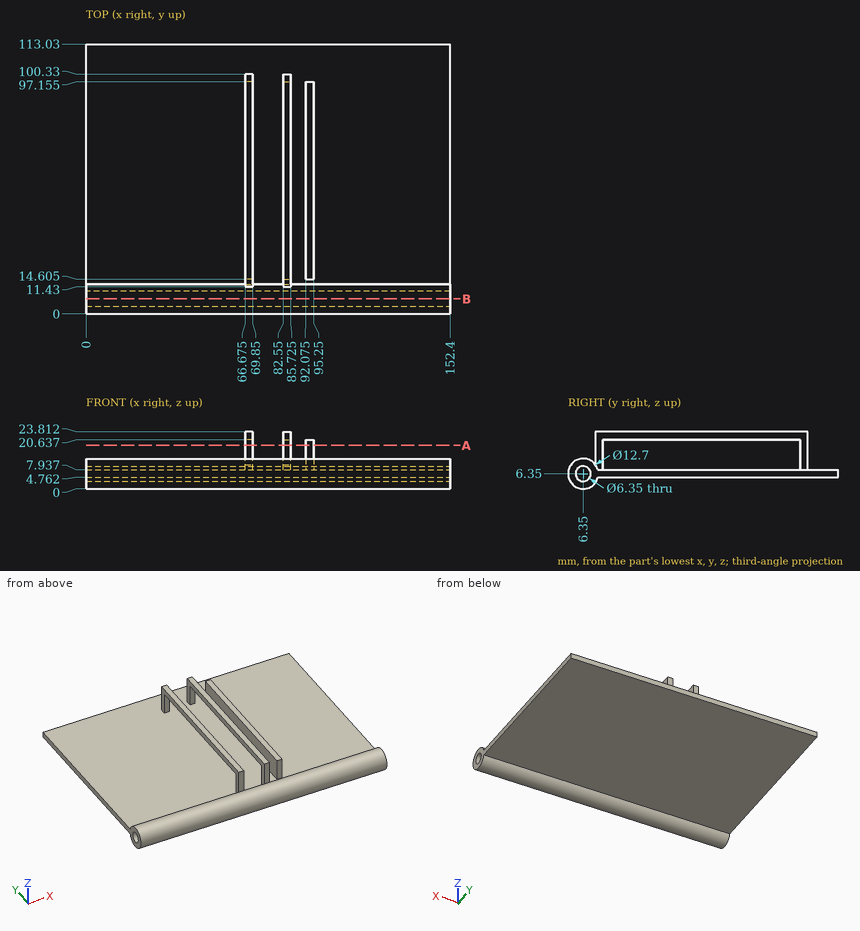
Job drawing, mm, ordinate dimensions from the low corner. One solid piece. Give positions to 0.01 mm unless a question says otherwise; leave off trailing zeros. Write each loop counter-clockwise with the first axis right and the second up, starting at its lowest first coordinate (ties: lowest second). Pieces come first, ordered by that corner, then holes. Notation, with made-up numbers: (-12.75, 46) -> (11.25, 46) arc R13 ccw to (11.25, 66) -> close; hole circle Ø10 at (17.5, 9). An arc over 180 degrees is marked (long way). Return JSON: item names as keys, results as strings.
Item 1: Band-saw the part on B-B (y = 6.35). List the corners of the cut face in (x, z) (1 decimal).
Answer below:
{"outline": "(0, 0) -> (152.4, 0) -> (152.4, 3.2) -> (0, 3.2) -> close; (0, 9.5) -> (152.4, 9.5) -> (152.4, 12.7) -> (0, 12.7) -> close"}
Item 2: Drill centre lines: probe 1 along Z at (x, y) = (111.5, 6.35) (1 decimal); probe 2 along Z at (x, y) = (114.5, 79); probe 3 along Y at (x, z) = (75, 6) (1 decimal). Where is each one in solid material? Low to high.
Answer below:
{"probe 1": "z = 0 to 3.2, 9.5 to 12.7", "probe 2": "z = 4.76 to 7.94", "probe 3": "y = 0 to 3.2, 9.5 to 113"}
Item 3: Drop flat-ended pins along their axis: pin 1 (1.6 mm diameter, centred on x = 83.5, z = 19.5, fed in from +Y); pin 2 (2 mm diameter, centred on x = 53.5, y = 40, fed in from -Z); pin 3 (6 mm diameter, centred on x = 125.5, y = 67.5, fed in from +Z); pin 4 (12 mm diameter, centred on y = 77, z = 13.5, fed in from +X). Give the stop position or say it passes through.
Answer below:
{"pin 1": "stops at y = 100.33", "pin 2": "stops at z = 4.76", "pin 3": "stops at z = 7.94", "pin 4": "stops at x = 152.4"}
Item 4: Band-saw the part on A-A (z = 18.25). Give the number of separate pieces and of enclosed holes in the cut face.
Answer below:
{"separate pieces": "5", "enclosed holes": "0"}
